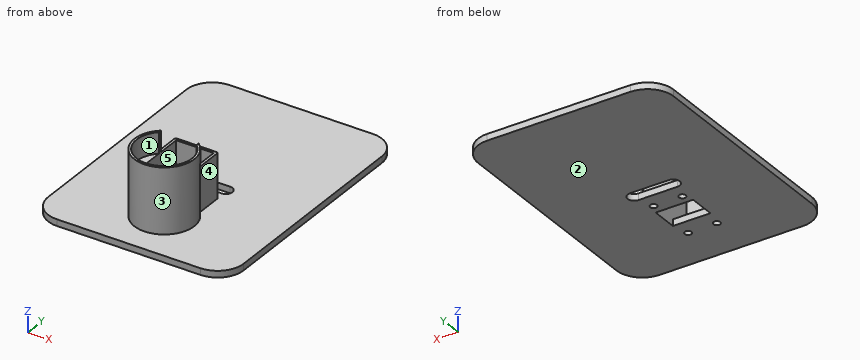
Autodesk Fusion 360 part; units mm, degrees
sketch "スケッチ1" plane through (0, 0, 0) normal (0, 0, 1) x (1, 0, 0)
  line L0 (20, 0) -> (130, 0)
  line L1 (150, 20) -> (150, 180)
  line L2 (130, 200) -> (20, 200)
  line L3 (0, 180) -> (0, 20)
  arc A0 (20, 200) -> (0, 180) centre (20, 180) ccw
  arc A1 (150, 180) -> (130, 200) centre (130, 180) ccw
  arc A2 (0, 20) -> (20, 0) centre (20, 20) ccw
  arc A3 (130, 0) -> (150, 20) centre (130, 20) ccw
  point P0 (150, 0)
  point P1 (0, 200)
  dimension "d1" = 150
  dimension "d2" = 200
  dimension "d5" = 20
  dimension "d6" = 20
  dimension "d7" = 20
  dimension "d8" = 20
extrude "押し出し1" add sketch "スケッチ1" along normal blind 5
sketch "スケッチ2" plane through (0, 0, 5) normal (0, 0, 1) x (-1, 0, 0)
  arc A0 (-130, 0) -> (-150, -20) centre (-130, -20) ccw
  arc A1 (-150, -180) -> (-130, -200) centre (-130, -180) ccw
  line L0 (-130, -200) -> (-20, -200)
  arc A2 (-20, -200) -> (0, -180) centre (-20, -180) ccw
  arc A3 (0, -20) -> (-20, 0) centre (-20, -20) ccw
  line L1 (-20, 0) -> (-130, 0)
  line L2 (-89.4, -30) -> (-60.6, -30)
  line L3 (-60.6, -30) -> (-60.6, -76.8)
  line L4 (-60.6, -76.8) -> (-89.4, -76.8)
  line L5 (-89.4, -76.8) -> (-89.4, -30)
  line L6 (-91.4, -28) -> (-58.6, -28)
  line L7 (-58.6, -28) -> (-58.6, -78.8)
  line L8 (-58.6, -78.8) -> (-91.4, -78.8)
  line L9 (-91.4, -78.8) -> (-91.4, -28)
  line L10 (0, -180) -> (0, -20)
  dimension "d9" = 28.8
  dimension "d10" = 46.8
  dimension "d11" = 150
  dimension "d12" = 200
  dimension "d13" = 60.6
  dimension "d14" = 30
  dimension "d15" = 32.8
  dimension "d16" = 50.8
  dimension "d17" = 58.6
  dimension "d18" = 28
extrude "押し出し2" add sketch "スケッチ2" along normal blind 34
sketch "スケッチ3" plane through (0, 0, 39) normal (0, 0, 1) x (-1, 0, 0)
  line L0 (-60.6, -76.8) -> (-89.4, -76.8)
  line L1 (-89.4, -76.8) -> (-89.4, -30)
  line L2 (-89.4, -30) -> (-60.6, -30)
  line L3 (-60.6, -30) -> (-60.6, -76.8)
  line L4 (-91.4, -78.8) -> (-58.6, -78.8)
  line L5 (-58.6, -78.8) -> (-58.6, -28)
  line L6 (-58.6, -28) -> (-91.4, -28)
  line L7 (-91.4, -28) -> (-91.4, -78.8)
  circle A0 centre (-75, -41.3) radius 21.25
  circle A1 centre (-75, -41.3) radius 23
  dimension "d21" = 42.5
  dimension "d22" = 11.3
  dimension "d23" = 46
extrude "押し出し3" add sketch "スケッチ3" against normal blind 2 contours L5 L6 L7 A0
extrude "押し出し4" add sketch "スケッチ3" along normal blind 16 and the other way blind 34 contours L3 L5 A0 A1 | L1 L7 A0 A1 | L5 L7 A0 A1
fillet "フィレット1" radius 1 1 edges at (91.4, 78.8, 22)
fillet "フィレット2" radius 1 1 edges at (58.6, 78.8, 22)
sketch "スケッチ4" plane through (0, 0, 5) normal (0, 0, 1) x (-1, 0, 0)
  line L0 (-60.6, -76.8) -> (-60.6, -30)
  line L1 (-60.6, -30) -> (-89.4, -30)
  line L2 (-89.4, -30) -> (-89.4, -76.8)
  line L3 (-89.4, -76.8) -> (-60.6, -76.8)
  line L4 (-89.4, -46) -> (-60.6, -46)
  line L5 (-60.6, -46) -> (-60.6, -66)
  line L6 (-60.6, -66) -> (-89.4, -66)
  line L7 (-89.4, -66) -> (-89.4, -46)
  dimension "d35" = 16
  dimension "d36" = 20
extrude "押し出し5" cut sketch "スケッチ4" against normal up to surface (5 mm away) contours L0 L2 L4 L5 L6 L7
sketch "スケッチ5" plane through (0, 0, 0) normal (0, 0, -1) x (1, 0, 0)
  line L0 (89.4, -46) -> (89.4, -66)
  line L1 (89.4, -66) -> (60.6, -66)
  line L2 (60.6, -66) -> (60.6, -46)
  line L3 (60.6, -46) -> (89.4, -46)
  arc A0 (150, -20) -> (130, 0) centre (130, -20) ccw
  line L4 (130, 0) -> (20, 0)
  arc A1 (20, 0) -> (0, -20) centre (20, -20) ccw
  line L5 (0, -20) -> (0, -180)
  arc A2 (0, -180) -> (20, -200) centre (20, -180) ccw
  line L6 (20, -200) -> (130, -200)
  arc A3 (130, -200) -> (150, -180) centre (130, -180) ccw
  line L7 (150, -180) -> (150, -20)
  circle A4 centre (64, -33.4) radius 2.6
  circle A5 centre (86, -73.4) radius 2.6
  circle A6 centre (86, -33.4) radius 2.6
  circle A7 centre (64, -73.4) radius 2.6
  line L8 (75, -25) -> (75, -85)
  line L9 (89.4, -30) -> (60.6, -30)
  line L10 (60.6, -76.8) -> (89.4, -76.8)
  circle A8 centre (64, -33.4) radius 1.4
  circle A9 centre (86, -33.4) radius 1.4
  circle A10 centre (64, -73.4) radius 1.4
  circle A11 centre (86, -73.4) radius 1.4
  dimension "d39" = 5.2
  dimension "d40" = 5.2
  dimension "d41" = 5.2
  dimension "d42" = 5.2
  dimension "d43" = 22
  dimension "d44" = 22
  dimension "d45" = 40
  dimension "d46" = 40
  dimension "d47" = 75
  dimension "d48" = 11
  dimension "d49" = 11
  dimension "d50" = 46.8
  dimension "d51" = 3.4
  dimension "d52" = 3.4
  dimension "d53" = 2.8
  dimension "d54" = 2.8
  dimension "d55" = 2.8
  dimension "d56" = 2.8
extrude "押し出し6" cut sketch "スケッチ5" against normal blind 5 contours A8 | A9 | A10 | A11
extrude "押し出し7" cut sketch "スケッチ5" against normal blind 4 contours A4 | A5 | A6 | A7
sketch "スケッチ6" plane through (0, 0, 5) normal (0, 0, 1) x (-1, 0, 0)
  arc A0 (-58.6, -57.4258) -> (-91.4, -57.4258) centre (-75, -41.3) ccw
  line L0 (-58.6, -57.4258) -> (-58.6, -77.8)
  arc A1 (-59.6, -78.8) -> (-58.6, -77.8) centre (-59.6, -77.8) ccw
  line L1 (-59.6, -78.8) -> (-90.4, -78.8)
  arc A2 (-91.4, -77.8) -> (-90.4, -78.8) centre (-90.4, -77.8) ccw
  line L2 (-91.4, -77.8) -> (-91.4, -57.4258)
  arc A3 (-130, 0) -> (-150, -20) centre (-130, -20) ccw
  line L3 (-150, -20) -> (-150, -180)
  arc A4 (-150, -180) -> (-130, -200) centre (-130, -180) ccw
  line L4 (-130, -200) -> (-20, -200)
  arc A5 (-20, -200) -> (0, -180) centre (-20, -180) ccw
  line L5 (0, -180) -> (0, -20)
  arc A6 (0, -20) -> (-20, 0) centre (-20, -20) ccw
  line L6 (-20, 0) -> (-130, 0)
  circle A7 centre (-90, -90) radius 5
  circle A8 centre (-60, -90) radius 5
  line L7 (-90, -85) -> (-60, -85)
  line L8 (-60, -85) -> (-60, -95)
  line L9 (-60, -95) -> (-90, -95)
  line L10 (-90, -95) -> (-90, -85)
  dimension "d61" = 10
  dimension "d62" = 10
extrude "押し出し8" cut sketch "スケッチ6" against normal blind 5 contours A7 L10 | A7 A8 L7 L9 | A7 L10 | A8 L8 | A8 L8
equation "d13 = ( 150 mm - d9 ) / 2"
equation "d15 = d9 + 4 mm"
equation "d16 = d10 + 4 mm"
equation "d17 = ( d11 - d15 ) / 2"
equation "d18 = d14 - 2 mm"
equation "d44 = d43"
equation "d46 = d45"
equation "d48 = d43 / 2"
equation "d49 = d48"
equation "d51 = ( d50 - d45 ) / 2"
equation "d52 = d51"
Design review of the part built by this model. Coordinates are the model's own, in mm. Face numbers are marked on the shaded views. A direction names the side the tool comes from. Give positions to 0.01 mm unless a question says otherwise; leave off trailing zeros. Write each loop counter-clockwise with the first axis right and the second up, starting at its lowest first coordinate (ties: lowest second). Pieces come first, ordered by that corner, then holes. Notation, with made-up numbers: M 87.5,54.25 L 128.5,54.25 A37 cw 128.5,93.25 Z; hole C -30,-20.75 d4. An arc over 180 degrees is marked long. Answer as a JSON object with one key per item and string values. Group by question number.
1) For line 1 along X through (y, z) = (73.4, 2.45); line 2 along X through (y, z) = (33.4, 4.4); line 3 along Y through (x, z) = (86, 1.95), list the stretches that pass through material, from the lowest coordinate up.
2) Mouldability with a two-part tool opening along Y and no side actions: class the marked faces 1, 2 and 3 as released by +Y, released by -Y, zero draft, split by the parting line, or undercut.
3) Tool access review of the marked faces 4 and 5: name each direction out of +Z, -Z, +X, -X, +Y, -Y from which nothing blocks a thin tool from reaching the whole face with its end or side.
4) We need section A-A (y = 41.3). Give the boundary of the cut face in (x, z).
5) Clearance check with flat-ended pins moving along their axes: pin 1 Ø8 at (y, z) = (46, 26.5) entering from +X; pin 2 Ø16 at (x, z) = (72, 21) entering from -Y; pin 3 Ø17 at (x, y) = (73.5, 72.5) entering from +Z. State where each tip first meets the part, or that it passes through.
6) We need section D-D (y = 90). Give the boundary of the cut face in (x, z), and give its area (3 significant figures).
7) We need section C-C (z = 29). Give the boundary of the cut face in (x, y).
8) We need section B-B (x = 77). Give the boundary of the cut face in (y, z).
Answer key:
{
 "1": {"line 1": "x = 0 to 61.4, 66.6 to 83.4, 88.6 to 150", "line 2": "x = 0 to 62.6, 65.4 to 84.6, 87.4 to 150", "line 3": "y = 0 to 30.8, 36 to 46, 66 to 70.8, 76 to 85, 95 to 200"},
 "2": {"face 1": "undercut", "face 2": "zero draft", "face 3": "split by the parting line"},
 "3": {"face 4": "+Z, +X, +Y", "face 5": "+Z"},
 "4": {"outline": "M 0,0 L 150,0 L 150,5 L 98,5 L 98,55 L 96.25,55 L 96.25,39 L 89.4,39 L 89.4,5 L 60.6,5 L 60.6,39 L 53.75,39 L 53.75,55 L 52,55 L 52,5 L 0,5 Z; hole M 53.75,5 L 58.6,5 L 58.6,37 L 53.75,37 Z; hole M 91.4,5 L 96.25,5 L 96.25,37 L 91.4,37 Z"},
 "5": {"pin 1": "stops at x = 97.99", "pin 2": "stops at y = 18.3", "pin 3": "stops at z = 39"},
 "6": {"outline": "M 0,0 L 55,0 L 55,5 L 0,5 Z; M 95,0 L 150,0 L 150,5 L 95,5 Z", "area": "550 mm²"},
 "7": {"outline": "M 58.6,57.43 A23 ccw long 91.4,57.43 L 91.4,77.8 A1 ccw 90.4,78.8 L 59.6,78.8 A1 ccw 58.6,77.8 Z; hole M 58.6,28 L 58.6,54.81 A21.25 ccw long 91.4,54.81 L 91.4,28 Z; hole M 60.6,30 L 89.4,30 L 89.4,76.8 L 60.6,76.8 Z"},
 "8": {"outline": "M 0,0 L 46,0 L 46,5 L 30,5 L 30,39 L 20.14,39 L 20.14,55 L 18.39,55 L 18.39,5 L 0,5 Z; M 66,0 L 85,0 L 85,5 L 78.8,5 L 78.8,39 L 76.8,39 L 76.8,5 L 66,5 Z; M 95,0 L 200,0 L 200,5 L 95,5 Z; hole M 20.14,5 L 28,5 L 28,37 L 20.14,37 Z"}
}
